Part model, mm, in its own coordinate system. Coordinates: 2 decimals unless noted, no trailing zeros. Order: outer loops, then holes, each group sorted by start corner. A loop starts at its lowest first (then second) coordinate and runs counter-clockwise, first axis right, second up.
1) Wall check: L1, parallel to Y at x = 35, z = 3.35; L2, parallel to X at y = 14.5, z = 2.15; L3, parallel to X at y = 12, z = 2.05. Give the ranges that are in metal, low to high.
2) Cut at A-A (y = 0). List the corners of the cut face in (x, z), and give its area (3 significant figures).
3) Cut at C-C (y = 13.48). List the corners of the cut face in (x, z).
4) Cut at B-B (x = -35). List the corners of the cut face in (y, z).
```python
from build123d import *

# Parameters (mm, degrees)
SKETCH1_W           = 101.6
SKETCH1_H           = 43.04
BOSS_EXTRUDE1_DEPTH = 5
SKETCH2_R           = 2.5
CUT_EXTRUDE1_DEPTH  = 56.396303126
SKETCH3_R           = 2
CUT_EXTRUDE2_DEPTH  = 56.396303126


with BuildPart() as part:
    # Sketch1 → Boss-Extrude1 (new body)
    with BuildSketch(Plane.XY):
        Rectangle(SKETCH1_W, SKETCH1_H)
    extrude(amount=BOSS_EXTRUDE1_DEPTH)

    # Sketch2 → Cut-Extrude1 (cut, through all)
    with BuildSketch(Plane.XY.offset(5)):
        with Locations((16.93333334, 0)):
            Circle(SKETCH2_R)
    extrude(amount=-CUT_EXTRUDE1_DEPTH, mode=Mode.SUBTRACT)

    # Sketch3 → Cut-Extrude2 (cut, through all)
    with BuildSketch(Plane.XY.offset(5)):
        with Locations((-35, 13.48)):
            Circle(SKETCH3_R)
        with Locations((35, 13.48)):
            Circle(SKETCH3_R)
    extrude(amount=-CUT_EXTRUDE2_DEPTH, mode=Mode.SUBTRACT)


solid = part.part
```
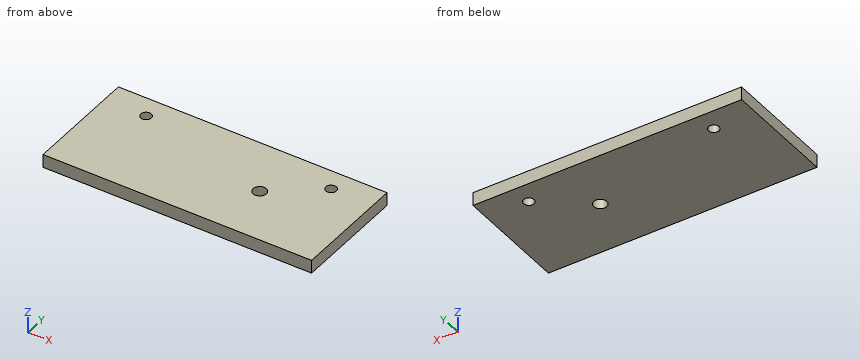
Geometry check:
1. L1: y = -21.52 to 11.48, 15.48 to 21.52
1. L2: x = -50.8 to -36.72, -33.28 to 33.28, 36.72 to 50.8
1. L3: x = -50.8 to -36.35, -33.65 to 33.65, 36.35 to 50.8
2. outline: (-50.8, 0) - (14.43, 0) - (14.43, 5) - (-50.8, 5) - close; (19.43, 0) - (50.8, 0) - (50.8, 5) - (19.43, 5) - close
2. area: 483 mm2
3. outline: (-50.8, 0) - (-37, 0) - (-37, 5) - (-50.8, 5) - close; (-33, 0) - (33, 0) - (33, 5) - (-33, 5) - close; (37, 0) - (50.8, 0) - (50.8, 5) - (37, 5) - close
4. outline: (-21.52, 0) - (11.48, 0) - (11.48, 5) - (-21.52, 5) - close; (15.48, 0) - (21.52, 0) - (21.52, 5) - (15.48, 5) - close
